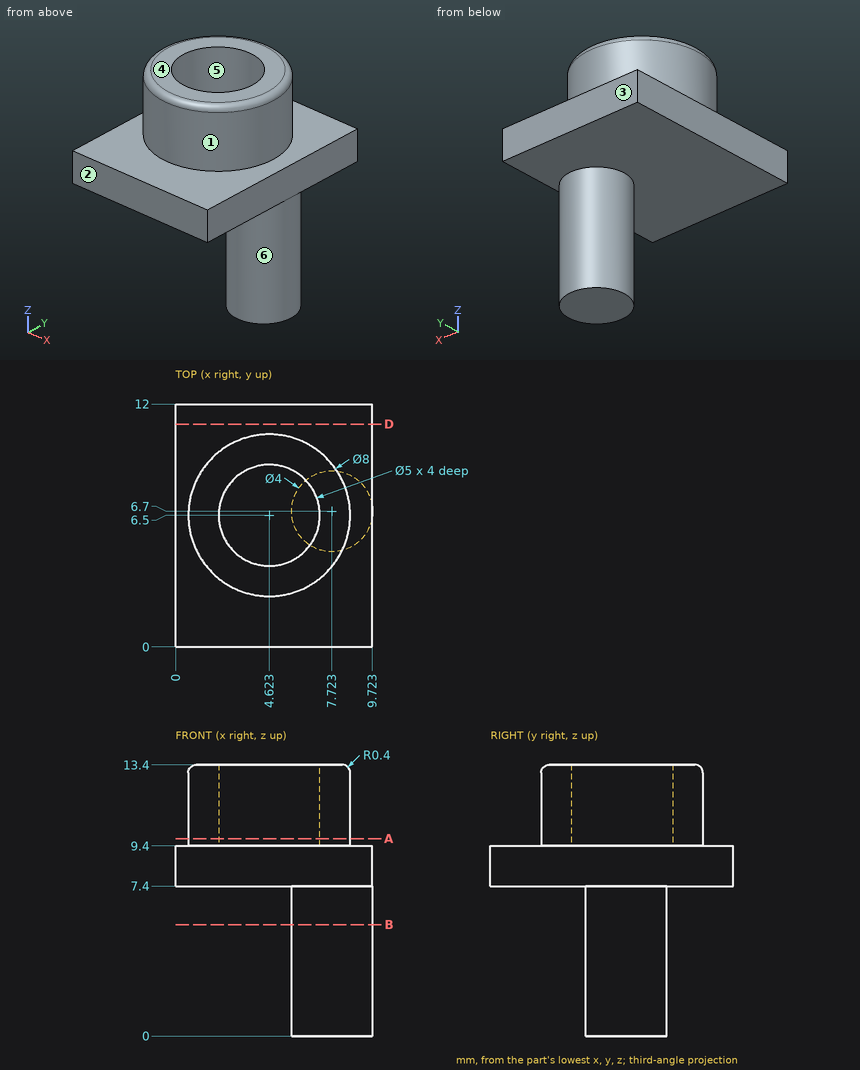
Geometry check sheet. Reference: drawing and pictorial views, mm from the part's lowest x, y, z. A direction names the side the tool comes from. Give positions to 0.01 mm unless a question says otherwise; leave off trailing zeros. Write each loop counter-clockwise with the first axis right and the second up, starting at its lowest first coordinate (ties: lowest second). Pieces come first, ordered by that corner, then holes.
Item 1: Cross-section at B-B (z = 5.5). Enter the section's corners in (x, y), and give its area (3 significant figures).
Item 2: Access from +Z, -Z, +X, -X, +Y, -Y to the whole of each face (thin tool, end or side, straight path). Record for the marked faces 1 and 2.
Item 3: Draft check along Y on the marked faces 3, 4, 5 and 6. Enter one of: released by +Y, released by -Y, zero draft, split by the parting line, or undercut.
Item 4: Gauge pin test, flat ends, axial feed: pin 1 (1 mm diameter, centred on x = 2, y = 9.5, fed in from +Z); pin 2 (4 mm diameter, centred on x = 5, y = 6.5, fed in from +Z); pin 3 (2 mm diameter, centred on y = 5, z = 5.5, fed in from -X). Record the tip position at first contact, or that the pin passes through.
Item 5: Cross-section at A-A (z = 9.75). Enter the section's corners in (x, y).
Item 6: Cross-section at D-D (y = 11). Enter the section's corners in (x, z).
Item 7: Scan lines: L1, parallel to Z at x = 6, y = 3.75; L2, parallel to Z at x = 3, y = 6.25; L3, parallel to X at y = 5.25, z = 12.5. Record each from-to range of solid material in increasing order.
Report:
1. outline: circle Ø4 at (7.72, 6.7)
1. area: 12.6 mm2
2. face 1: +Z
2. face 2: +Z, -Z, +X, -X, -Y
3. face 3: released by +Y
3. face 4: zero draft
3. face 5: undercut
3. face 6: split by the parting line
4. pin 1: stops at z = 13.4
4. pin 2: stops at z = 9.4
4. pin 3: stops at x = 5.85
5. outline: circle Ø8 at (4.62, 6.5); hole circle Ø5 at (4.62, 6.5)
6. outline: (0, 7.4) - (9.72, 7.4) - (9.72, 9.4) - (0, 9.4) - close
7. L1: z = 7.4 to 13.4
7. L2: z = 7.4 to 9.4
7. L3: x = 0.82 to 2.46, 6.79 to 8.42
